Verification items for the finished model (mm, model axes). Round coordinates to 2 decimals unless told otherwise and drop trailing zeros. Write each loop counter-clockwise with the first axis right and the second up, starting at its lowest first coordinate (ties: lowest second). Pieces come first, ordered by that corner, then holes. Notation, with made-up numbers: M 11.25,39.5 L 40.25,39.5 A30 ccw 40.25,62.5 Z; hole C 10,24 d6. An arc over 180 degrees is marked long. One line per question, with ' | ' between items.
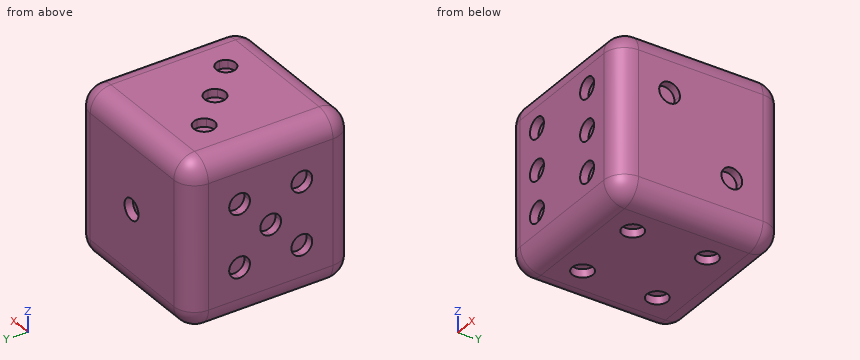
from build123d import *

# Parameters (mm, degrees)
F0_W      = 50.8
F0_H      = 50.8
F1_DEPTH  = 50.8
F2_R      = 6.35
F3_R      = 3.175
F4_DEPTH  = 2.54
F6_DEPTH  = 2.54
F8_DEPTH  = 2.54
F10_DEPTH = 2.54
F12_DEPTH = 2.54
F14_DEPTH = 2.54


with BuildPart() as f1:
    # F0 (on Top) → F1 (new body)
    with BuildSketch(Plane.XY):
        with Locations((-0.2253249615, 17.7784047042)):
            Rectangle(F0_W, F0_H)
    extrude(amount=F1_DEPTH)

    # F2
    f2_edges = [f1.edges().sort_by_distance(p)[0] for p in [
        (-25.625325, -7.621595, 25.4),
        (25.174675, -7.621595, 25.4),
        (-0.225325, -7.621595, 0),
        (-0.225325, -7.621595, 50.8),
        (25.174675, 43.178405, 25.4),
        (25.174675, 17.778405, 0),
        (-25.625325, 43.178405, 25.4),
        (25.174675, 17.778405, 50.8),
        (-0.225325, 43.178405, 0),
        (-25.625325, 17.778405, 0),
        (-25.625325, 17.778405, 50.8),
        (-0.225325, 43.178405, 50.8),
    ]]
    fillet(f2_edges, radius=F2_R)

    # F3 (on face) → F4 (cut)
    with BuildSketch(Plane(origin=(0, 43.1784047042, 0), x_dir=(-1, 0, 0), z_dir=(0, 1, 0))):
        with Locations((0, 25.4)):
            Circle(F3_R)
    extrude(amount=-F4_DEPTH, mode=Mode.SUBTRACT)

    # F5 (on face) → F6 (cut)
    with BuildSketch(Plane.XZ.offset(7.6215952958)):
        with BuildLine():
            Line((-11.6553249615, 34.925), (-11.6553249615, 41.275))
            ThreePointArc((-11.6553249615, 41.275), (-14.8303249615, 38.1), (-11.6553249615, 34.925))
        make_face()
        with BuildLine():
            ThreePointArc((-8.4803249615, 38.1), (-9.4102609313, 40.3450640303), (-11.6553249615, 41.275))
            Line((-11.6553249615, 41.275), (-11.6553249615, 34.925))
            ThreePointArc((-11.6553249615, 34.925), (-9.4102609313, 35.8549359697), (-8.4803249615, 38.1))
        make_face()
        with BuildLine():
            ThreePointArc((-8.4803249615, 25.4), (-9.4102609313, 27.6450640303), (-11.6553249615, 28.575))
            Line((-11.6553249615, 28.575), (-11.6553249615, 22.225))
            ThreePointArc((-11.6553249615, 22.225), (-9.4102609313, 23.1549359697), (-8.4803249615, 25.4))
        make_face()
        with BuildLine():
            Line((-11.6553249615, 22.225), (-11.6553249615, 28.575))
            ThreePointArc((-11.6553249615, 28.575), (-14.8303249615, 25.4), (-11.6553249615, 22.225))
        make_face()
        with BuildLine():
            Line((-11.6553249615, 15.875), (-11.6553249615, 9.525))
            ThreePointArc((-11.6553249615, 9.525), (-9.4102609313, 10.4549359697), (-8.4803249615, 12.7))
            ThreePointArc((-8.4803249615, 12.7), (-9.4102609313, 14.9450640303), (-11.6553249615, 15.875))
        make_face()
        with BuildLine():
            ThreePointArc((-11.6553249615, 15.875), (-14.8303249615, 12.7), (-11.6553249615, 9.525))
            Line((-11.6553249615, 9.525), (-11.6553249615, 15.875))
        make_face()
        with BuildLine():
            Line((11.2046750385, 15.875), (11.2046750385, 9.525))
            ThreePointArc((11.2046750385, 9.525), (13.4497390687, 10.4549359697), (14.3796750385, 12.7))
            ThreePointArc((14.3796750385, 12.7), (13.4497390687, 14.9450640303), (11.2046750385, 15.875))
        make_face()
        with BuildLine():
            ThreePointArc((11.2046750385, 15.875), (8.0296750385, 12.7), (11.2046750385, 9.525))
            Line((11.2046750385, 9.525), (11.2046750385, 15.875))
        make_face()
        with BuildLine():
            ThreePointArc((14.3796750385, 25.4), (13.4497390687, 27.6450640303), (11.2046750385, 28.575))
            Line((11.2046750385, 28.575), (11.2046750385, 22.225))
            ThreePointArc((11.2046750385, 22.225), (13.4497390687, 23.1549359697), (14.3796750385, 25.4))
        make_face()
        with BuildLine():
            Line((11.2046750385, 22.225), (11.2046750385, 28.575))
            ThreePointArc((11.2046750385, 28.575), (8.0296750385, 25.4), (11.2046750385, 22.225))
        make_face()
        with BuildLine():
            ThreePointArc((14.3796750385, 38.1), (13.4497390687, 40.3450640303), (11.2046750385, 41.275))
            Line((11.2046750385, 41.275), (11.2046750385, 34.925))
            ThreePointArc((11.2046750385, 34.925), (13.4497390687, 35.8549359697), (14.3796750385, 38.1))
        make_face()
        with BuildLine():
            Line((11.2046750385, 34.925), (11.2046750385, 41.275))
            ThreePointArc((11.2046750385, 41.275), (8.0296750385, 38.1), (11.2046750385, 34.925))
        make_face()
    extrude(amount=-F6_DEPTH, mode=Mode.SUBTRACT)

    # F7 (on face) → F8 (cut)
    with BuildSketch(Plane(origin=(-25.6253249615, 0, 0), x_dir=(0, -1, 0), z_dir=(-1, 0, 0))):
        with BuildLine():
            ThreePointArc((-24.1284047042, 34.925), (-25.0583406739, 37.1700640303), (-27.3034047042, 38.1))
            Line((-27.3034047042, 38.1), (-27.3034047042, 31.75))
            ThreePointArc((-27.3034047042, 31.75), (-25.0583406739, 32.6799359697), (-24.1284047042, 34.925))
        make_face()
        with BuildLine():
            Line((-27.3034047042, 31.75), (-27.3034047042, 38.1))
            ThreePointArc((-27.3034047042, 38.1), (-30.4784047042, 34.925), (-27.3034047042, 31.75))
        make_face()
        with BuildLine():
            Line((-8.2534047042, 31.75), (-8.2534047042, 38.1))
            ThreePointArc((-8.2534047042, 38.1), (-11.4284047042, 34.925), (-8.2534047042, 31.75))
        make_face()
        with BuildLine():
            ThreePointArc((-5.0784047042, 34.925), (-6.0083406739, 37.1700640303), (-8.2534047042, 38.1))
            Line((-8.2534047042, 38.1), (-8.2534047042, 31.75))
            ThreePointArc((-8.2534047042, 31.75), (-6.0083406739, 32.6799359697), (-5.0784047042, 34.925))
        make_face()
        with BuildLine():
            ThreePointArc((-14.6034047042, 25.4), (-15.5333406739, 27.6450640303), (-17.7784047042, 28.575))
            Line((-17.7784047042, 28.575), (-17.7784047042, 25.4))
            Line((-17.7784047042, 25.4), (-14.6034047042, 25.4))
        make_face()
        with BuildLine():
            Line((-14.6034047042, 25.4), (-17.7784047042, 25.4))
            Line((-17.7784047042, 25.4), (-17.7784047042, 22.225))
            ThreePointArc((-17.7784047042, 22.225), (-15.5333406739, 23.1549359697), (-14.6034047042, 25.4))
        make_face()
        with BuildLine():
            Line((-17.7784047042, 25.4), (-20.9534047042, 25.4))
            ThreePointArc((-20.9534047042, 25.4), (-20.0234687345, 23.1549359697), (-17.7784047042, 22.225))
            Line((-17.7784047042, 22.225), (-17.7784047042, 25.4))
        make_face()
        with BuildLine():
            ThreePointArc((-17.7784047042, 28.575), (-20.0234687345, 27.6450640303), (-20.9534047042, 25.4))
            Line((-20.9534047042, 25.4), (-17.7784047042, 25.4))
            Line((-17.7784047042, 25.4), (-17.7784047042, 28.575))
        make_face()
        with BuildLine():
            Line((-8.2534047042, 19.05), (-8.2534047042, 12.7))
            ThreePointArc((-8.2534047042, 12.7), (-6.0083406739, 13.6299359697), (-5.0784047042, 15.875))
            ThreePointArc((-5.0784047042, 15.875), (-6.0083406739, 18.1200640303), (-8.2534047042, 19.05))
        make_face()
        with BuildLine():
            ThreePointArc((-8.2534047042, 19.05), (-11.4284047042, 15.875), (-8.2534047042, 12.7))
            Line((-8.2534047042, 12.7), (-8.2534047042, 19.05))
        make_face()
        with BuildLine():
            ThreePointArc((-24.1284047042, 15.875), (-25.0583406739, 18.1200640303), (-27.3034047042, 19.05))
            Line((-27.3034047042, 19.05), (-27.3034047042, 12.7))
            ThreePointArc((-27.3034047042, 12.7), (-25.0583406739, 13.6299359697), (-24.1284047042, 15.875))
        make_face()
        with BuildLine():
            Line((-27.3034047042, 12.7), (-27.3034047042, 19.05))
            ThreePointArc((-27.3034047042, 19.05), (-30.4784047042, 15.875), (-27.3034047042, 12.7))
        make_face()
    extrude(amount=-F8_DEPTH, mode=Mode.SUBTRACT)

    # F9 (on face) → F10 (cut)
    with BuildSketch(Plane.YZ.offset(25.1746750385)):
        with BuildLine():
            ThreePointArc((30.4798430878, 15.8735616164), (28.5198629856, 18.8068791321), (25.0597790575, 18.1186256467))
            Line((25.0597790575, 18.1186256467), (29.5499071181, 13.6284975861))
            ThreePointArc((29.5499071181, 13.6284975861), (30.2381606035, 14.6585417186), (30.4798430878, 15.8735616164))
        make_face()
        with BuildLine():
            Line((29.5499071181, 13.6284975861), (25.0597790575, 18.1186256467))
            ThreePointArc((25.0597790575, 18.1186256467), (25.0597790575, 13.6284975861), (29.5499071181, 13.6284975861))
        make_face()
        with BuildLine():
            Line((10.4970303509, 32.6813743533), (6.0069022903, 37.1715024139))
            ThreePointArc((6.0069022903, 37.1715024139), (6.0069022903, 32.6813743533), (10.4970303509, 32.6813743533))
        make_face()
        with BuildLine():
            ThreePointArc((11.4269663206, 34.9264383836), (9.4669862183, 37.8597558993), (6.0069022903, 37.1715024139))
            Line((6.0069022903, 37.1715024139), (10.4970303509, 32.6813743533))
            ThreePointArc((10.4970303509, 32.6813743533), (11.1852838363, 33.7114184858), (11.4269663206, 34.9264383836))
        make_face()
    extrude(amount=-F10_DEPTH, mode=Mode.SUBTRACT)

    # F11 (on face) → F12 (cut)
    with BuildSketch(Plane(origin=(0, 0, 0), x_dir=(1, 0, 0), z_dir=(0, 0, -1))):
        with BuildLine():
            Line((8.0296750385, -6.3484047042), (14.3796750385, -6.3484047042))
            ThreePointArc((14.3796750385, -6.3484047042), (11.2046750385, -3.1734047042), (8.0296750385, -6.3484047042))
        make_face()
        with BuildLine():
            ThreePointArc((8.0296750385, -6.3484047042), (11.2046750385, -9.5234047042), (14.3796750385, -6.3484047042))
            Line((14.3796750385, -6.3484047042), (8.0296750385, -6.3484047042))
        make_face()
        with BuildLine():
            Line((8.0296750385, -29.2084047042), (14.3796750385, -29.2084047042))
            ThreePointArc((14.3796750385, -29.2084047042), (11.2046750385, -26.0334047042), (8.0296750385, -29.2084047042))
        make_face()
        with BuildLine():
            ThreePointArc((8.0296750385, -29.2084047042), (11.2046750385, -32.3834047042), (14.3796750385, -29.2084047042))
            Line((14.3796750385, -29.2084047042), (8.0296750385, -29.2084047042))
        make_face()
        with BuildLine():
            Line((-8.4803249615, -29.2084047042), (-14.8303249615, -29.2084047042))
            ThreePointArc((-14.8303249615, -29.2084047042), (-11.6553249615, -32.3834047042), (-8.4803249615, -29.2084047042))
        make_face()
        with BuildLine():
            ThreePointArc((-8.4803249615, -29.2084047042), (-11.6553249615, -26.0334047042), (-14.8303249615, -29.2084047042))
            Line((-14.8303249615, -29.2084047042), (-8.4803249615, -29.2084047042))
        make_face()
        with BuildLine():
            Line((-8.4803249615, -6.3484047042), (-14.8303249615, -6.3484047042))
            ThreePointArc((-14.8303249615, -6.3484047042), (-11.6553249615, -9.5234047042), (-8.4803249615, -6.3484047042))
        make_face()
        with BuildLine():
            ThreePointArc((-8.4803249615, -6.3484047042), (-11.6553249615, -3.1734047042), (-14.8303249615, -6.3484047042))
            Line((-14.8303249615, -6.3484047042), (-8.4803249615, -6.3484047042))
        make_face()
    extrude(amount=-F12_DEPTH, mode=Mode.SUBTRACT)

    # F13 (on face) → F14 (cut)
    with BuildSketch(Plane.XY.offset(50.8)):
        with BuildLine():
            Line((2.0197390687, 15.5333406739), (-2.4703889918, 20.0234687345))
            ThreePointArc((-2.4703889918, 20.0234687345), (-2.4703889918, 15.5333406739), (2.0197390687, 15.5333406739))
        make_face()
        with BuildLine():
            ThreePointArc((2.9496750385, 17.7784047042), (0.9896949362, 20.7117222199), (-2.4703889918, 20.0234687345))
            Line((-2.4703889918, 20.0234687345), (2.0197390687, 15.5333406739))
            ThreePointArc((2.0197390687, 15.5333406739), (2.7079925542, 16.5633848064), (2.9496750385, 17.7784047042))
        make_face()
        with BuildLine():
            ThreePointArc((-7.1214249615, 27.8495047042), (-9.0814050638, 30.7828222199), (-12.5414889918, 30.0945687345))
            Line((-12.5414889918, 30.0945687345), (-8.0513609313, 25.6044406739))
            ThreePointArc((-8.0513609313, 25.6044406739), (-7.3631074458, 26.6344848064), (-7.1214249615, 27.8495047042))
        make_face()
        with BuildLine():
            Line((-8.0513609313, 25.6044406739), (-12.5414889918, 30.0945687345))
            ThreePointArc((-12.5414889918, 30.0945687345), (-12.5414889918, 25.6044406739), (-8.0513609313, 25.6044406739))
        make_face()
        with BuildLine():
            Line((7.7587259792, 9.7943537635), (11.9328240977, 5.6202556449))
            ThreePointArc((11.9328240977, 5.6202556449), (12.5726360452, 6.5778018925), (12.7973081234, 7.7073047042))
            ThreePointArc((12.7973081234, 7.7073047042), (10.9752778502, 10.4341657109), (7.7587259792, 9.7943537635))
        make_face()
        with BuildLine():
            ThreePointArc((7.7587259792, 9.7943537635), (7.7587259792, 5.6202556449), (11.9328240977, 5.6202556449))
            Line((11.9328240977, 5.6202556449), (7.7587259792, 9.7943537635))
        make_face()
    extrude(amount=-F14_DEPTH, mode=Mode.SUBTRACT)


solid = f1.part
1. Go/stop test with flat-tipped pins: P1, Ø5, axis at x = 10.5, z = 25.5, coming from the -Y side; P2, Ø3, axis at x = -13, y = 6.5, coming from the -Z side; P3, Ø3, axis at x = -12.5, z = 12, coming from the -Y side; P4, Ø3, axis at y = 26.5, z = 15, coming from the +X side. Record where each tip stops, or that it passes through.
Results:
P1: stops at y = -7.62 | P2: stops at z = 2.54 | P3: stops at y = -5.08 | P4: stops at x = 22.63
2. Thickness scan on line 1 (Z direction, x = 0, y = 19.5); line 2 (X direction, y = 29, z = 6); line 3 (Z direction, x = 12.5, y = 7.5). Record the ranges inside material, lowest first.
Results:
line 1: z = 0 to 48.26 | line 2: x = -25.62 to 25.17 | line 3: z = 2.54 to 48.26
3. Section check B-B, the plane y = 17. Record the cut outline in (x, z).
Results:
outline: M -25.63,6.35 A6.35 ccw -19.28,0 L 18.82,0 A6.35 ccw 25.17,6.35 L 25.17,44.45 A6.35 ccw 18.82,50.8 L 2.85,50.8 L 2.85,48.26 L -3.3,48.26 L -3.3,50.8 L -19.28,50.8 A6.35 ccw -25.63,44.45 L -25.63,28.48 L -23.09,28.48 L -23.09,22.32 L -25.63,22.32 Z
4. Section check C-C, the plane z = 24. Record the cut outline in (x, y) (3 decimals).
Results:
outline: M -25.625,-1.272 A6.35 ccw -19.275,-7.622 L -14.505,-7.622 L -14.505,-5.082 L -8.806,-5.082 L -8.806,-7.622 L 8.355,-7.622 L 8.355,-5.082 L 14.054,-5.082 L 14.054,-7.622 L 18.825,-7.622 A6.35 ccw 25.175,-1.272 L 25.175,36.828 A6.35 ccw 18.825,43.178 L 2.85,43.178 L 2.85,40.638 L -2.85,40.638 L -2.85,43.178 L -19.275,43.178 A6.35 ccw -25.625,36.828 L -25.625,20.628 L -23.085,20.628 L -23.085,14.929 L -25.625,14.929 Z
5. Section check D-D, the plane x = -21. Record the cut outline in (y, z), then the cut area to 3 significant figures.
Results:
outline: M -7.38,6.35 A6.11 ccw -1.27,0.24 L 36.83,0.24 A6.11 ccw 42.94,6.35 L 42.94,44.45 A6.11 ccw 36.83,50.56 L -1.27,50.56 A6.11 ccw -7.38,44.45 Z | area: 2,500 mm2
